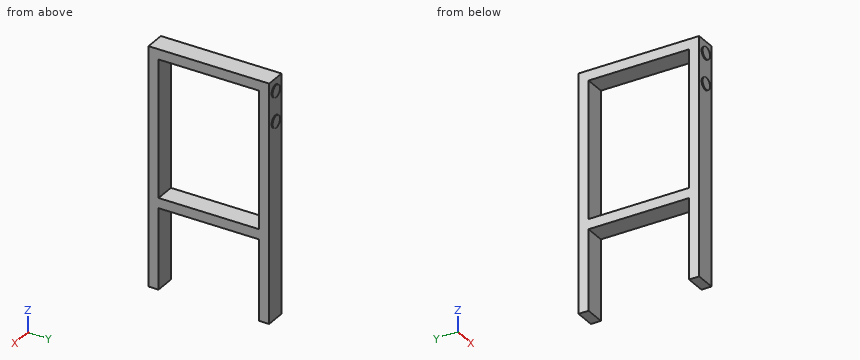
from build123d import *

# Parameters (mm, degrees)
F1_DEPTH = 12.7
F2_R     = 7.62
F3_DEPTH = 1.27


# Not quite as in the source:
# - a pattern or mirror of a feature is missing from the dataset's text; its kind, count and spacing are read off the source's solid


with BuildPart() as f1:
    # F0 (on Right) → F1 (new body, symmetric)
    with BuildSketch(Plane.YZ):
        Polygon((76.2, -149.86), (76.2, 149.86), (-76.2, 149.86), (-76.2, -149.86), (-63.5, -149.86), (-63.5, -48.26), (63.5, -48.26), (63.5, -149.86), align=None)
        Polygon((-63.5, 137.16), (0, 137.16), (63.5, 137.16), (63.5, -35.56), (-63.5, -35.56), align=None, mode=Mode.SUBTRACT)
    extrude(amount=F1_DEPTH, both=True)

    # F2 (on face) → F3 (join)
    with BuildSketch(Plane.XZ.offset(76.2)):
        with Locations((0, 96.52)):
            Circle(F2_R)
        with Locations((0, 134.62)):
            Circle(F2_R)
    f3 = extrude(amount=F3_DEPTH)

    # F3_copies: F3 across plane
    add(f3.mirror(Plane.ZX))


solid = f1.part
Can you work these out from the model? Positions are in its coordinate system, mm. Coordinates: 2 decimals unless noted, no trailing zeros. Loops run counter-clockwise (first coordinate to the right, second up) from the corner with the lowest first, then second, coordinate; pieces in that order, holes last. Notation, with made-up numbers: M 24.25,37.25 L 37.25,37.25 A10 ccw 37.25,46.25 Z; hole C -30,44 d1. An arc over 180 degrees is marked long. Return JSON: item names as keys, results as strings. Group by question number.
Item 1: I'm going to push flat-ended pins straight in: pin 1 Ø12.5 at (x, y) = (-5, -31.5) entering from -Z; pin 2 Ø8 at (x, z) = (-8, 31.5) entering from -Y; pin 3 Ø10 at (x, z) = (0.5, -6) entering from +Y. Where does each tip first touch, or does it pass through?
Item 2: Imagine slicing it at B-B (z = 54). Please give me the cut outline in (x, y).
Item 3: If I drill on L1, parallel to Z at x = -5.25, y = -11; L2, parallel to Y at x = -4, z = 135; L3, parallel to Y at x = 11.75, z = 41, over which ranges is the centre line in solid material (lowest first)? Write a range as from..to.
Item 4: Imagine slicing it at A-A (y = -26). Please give me the cut outline in (x, z).
Item 5: Imagine slicing it at D-D (z = 96.52). Please give me the cut outline in (x, y), and give its area (3 significant figures).
Verdict:
{
 "1": {"pin 1": "stops at z = -48.26", "pin 2": "stops at y = -76.2", "pin 3": "stops at y = 76.2"},
 "2": {"outline": "M -12.7,-76.2 L 12.7,-76.2 L 12.7,-63.5 L -12.7,-63.5 Z; M -12.7,63.5 L 12.7,63.5 L 12.7,76.2 L -12.7,76.2 Z"},
 "3": {"L1": "z = -48.26..-35.56, 137.16..149.86", "L2": "y = -77.47..-63.5, 63.5..77.47", "L3": "y = -76.2..-63.5, 63.5..76.2"},
 "4": {"outline": "M -12.7,-48.26 L 12.7,-48.26 L 12.7,-35.56 L -12.7,-35.56 Z; M -12.7,137.16 L 12.7,137.16 L 12.7,149.86 L -12.7,149.86 Z"},
 "5": {"outline": "M -12.7,-76.2 L -7.62,-76.2 L -7.62,-77.47 L 7.62,-77.47 L 7.62,-76.2 L 12.7,-76.2 L 12.7,-63.5 L -12.7,-63.5 Z; M -12.7,63.5 L 12.7,63.5 L 12.7,76.2 L 7.62,76.2 L 7.62,77.47 L -7.62,77.47 L -7.62,76.2 L -12.7,76.2 Z", "area": "684 mm^2"}
}
